Build history of the part. All positions in model axes, mm. Face numbers are marked on the shaded views. Round coordinates to 2 decimals unless told otherwise and drop trailing zeros. Order: outer loops, then holes, each group sorted by start corner. A loop starts at its lowest first (then second) coordinate and runs counter-clockwise, first axis right, second up. Notation, with made-up numbers: M -9.5,84 L 9.5,84 A24 ccw 9.5,99 Z; hole C 60.5,19.5 d6. An arc over 180 degrees is marked long. One line per item, written item: value. Start each with the question number.
Item 1: Probe L1, parallel to Z at x = -8, y = 8; L2, parallel to X at y = 4, z = -3.5; L3, parallel to X at y = 6.5, z = -1.25. List the from-to ranges inside material, lowest first.
Item 2: Band-saw the part on B-B, the plane z = -6.25. Write the cut outline in (x, y) (3 decimals), then the cut area to 3 significant figures.
Item 3: Two-plate mould, pull along X, no slides. Class the marked faces 1, 2, 3 and 4: +X half, -X half, draft (parallel to the pull), parting line (faces both ways), or undercut.
Item 4: Band-saw the part on A-A, the plane x = 40.64. Write the cut outline in (y, z) (3 decimals), then the cut area to 3 significant figures.
Item 5: Pin check, flat tips, straight feed: pin 1 (4 mm diameter, centred on y = 3.5, z = -5, fed in from +X); pin 2 (8 mm diameter, centred on x = 37, z = -5, fed in from -Y) (3 decimals). Stop position of each tip, or through.
Item 6: Band-saw the part on C-C, the plane y = 6.35. Write the cut outline in (x, z) (3 decimals), then the cut area to 3 significant figures.
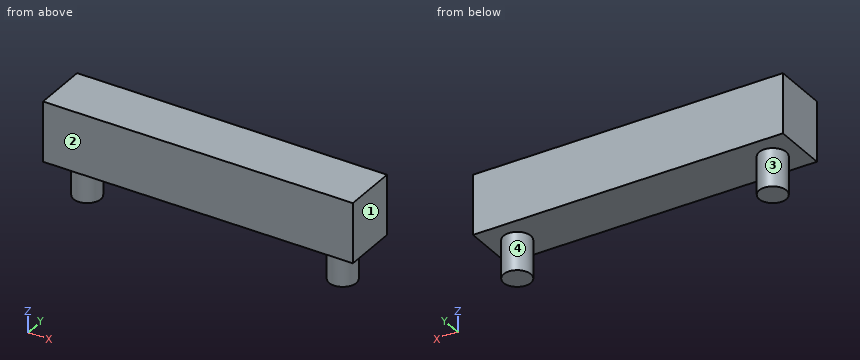
```python
from build123d import *

# Parameters (mm, degrees)
F0_W     = 25.4
F0_H     = 12.7
F0_W_2   = 46.99
F1_DEPTH = 7.62
F3_DEPTH = 8.89
F4_DEPTH = 6.35


with BuildPart() as f1:
    # F0 (on Top) → F1 (new body)
    with BuildSketch(Plane.XY):
        with Locations((-12.7, 6.35)):
            Rectangle(F0_W, F0_H)
        with Locations((23.495, 6.35)):
            Rectangle(F0_W_2, F0_H)
    extrude(amount=F1_DEPTH)

    # F2 (on face) → F3 (join)
    with BuildSketch(Plane(origin=(0, 0, 0), x_dir=(1, 0, 0), z_dir=(0, 0, -1))):
        with BuildLine():
            ThreePointArc((-15.875, -6.35), (-19.05, -3.175), (-22.225, -6.35))
            Line((-22.225, -6.35), (-19.05, -6.35))
            Line((-19.05, -6.35), (-15.875, -6.35))
        make_face()
        with BuildLine():
            Line((-19.05, -6.35), (-22.225, -6.35))
            ThreePointArc((-22.225, -6.35), (-19.05, -9.525), (-15.875, -6.35))
            Line((-15.875, -6.35), (-19.05, -6.35))
        make_face()
        with BuildLine():
            Line((40.64, -6.35), (43.815, -6.35))
            ThreePointArc((43.815, -6.35), (40.64, -3.175), (37.465, -6.35))
            Line((37.465, -6.35), (40.64, -6.35))
        make_face()
        with BuildLine():
            ThreePointArc((37.465, -6.35), (40.64, -9.525), (43.815, -6.35))
            Line((43.815, -6.35), (40.64, -6.35))
            Line((40.64, -6.35), (37.465, -6.35))
        make_face()
    extrude(amount=F3_DEPTH)

    # F4 (add): a face of the model
    f4_faces = [f1.faces().sort_by_distance(p)[0] for p in [
        (10.795, 6.35, 7.62),
    ]]
    extrude(f4_faces, amount=F4_DEPTH)


solid = f1.part
```
Output:
1. L1: z = 0 to 13.97
1. L2: x = -21.18 to -16.92, 38.51 to 42.77
1. L3: x = -22.22 to -15.88, 37.47 to 43.81
2. outline: C -19.05,6.35 d6.35; C 40.64,6.35 d6.35
2. area: 63.3 mm²
3. face 1: +X half
3. face 2: draft
3. face 3: undercut
3. face 4: undercut
4. outline: M 0,0 L 3.175,0 L 3.175,-8.89 L 9.525,-8.89 L 9.525,0 L 12.7,0 L 12.7,13.97 L 0,13.97 Z
4. area: 234 mm²
5. pin 1: stops at x = 43.7
5. pin 2: stops at y = 3.175
6. outline: M -25.4,0 L -22.225,0 L -22.225,-8.89 L -15.875,-8.89 L -15.875,0 L 37.465,0 L 37.465,-8.89 L 43.815,-8.89 L 43.815,0 L 46.99,0 L 46.99,13.97 L -25.4,13.97 Z
6. area: 1,120 mm²
